The model under review builds one solid part; all positions refer to its coordinate system, in mm. A direction names the side the tool comes from. Coordinates: 2 decimals unless noted, no trailing zeros. Order: outer loops, then holes, each group sorted by start corner. A loop starts at its lowest first (then second) coordinate and runs counter-clockwise, first axis right, second up. Notation, with made-up numbers: (80.5, -28) -> (95.5, -28) arc R15 cw to (95.5, -10) -> close; hole circle Ø11 at (85, 44.25). An arc over 180 degrees is marked (long way). Use one line per item in the form item = value.
from build123d import *

# Parameters (mm, degrees)
F0_R     = 19
F0_R_2   = 17.5
F1_DEPTH = 30
F5_DEPTH = 2
F7_DEPTH = 8
F8_W     = 3.0304512245
F8_H     = 4
F8_W_2   = 3.9695487755
F9_DEPTH = 25


# Not quite as in the source:
# - a feature names something its author has since deleted; it is built from what else it names


with BuildPart() as f1:
    # F0 (on Top) → F1 (new body)
    with BuildSketch(Plane.XY):
        Circle(F0_R)
        Circle(F0_R_2, mode=Mode.SUBTRACT)
    extrude(amount=F1_DEPTH)

    # F2 (on Front) → F3 (revolve)
    with BuildSketch(Plane.XZ):
        with BuildLine():
            Line((0, 41.805047949), (0, 30))
            Line((0, 30), (19, 30))
            ThreePointArc((19, 30), (13.3813344534, 37.450646936), (5.1278058683, 41.805047949))
            Line((5.1278058683, 41.805047949), (0, 41.805047949))
        make_face()
    revolve(axis=Axis((0, 0, 35.9025239745), (0, 0, 1)))

    # F4 (on Top) → F5 (join)
    with BuildSketch(Plane.XY):
        with BuildLine():
            ThreePointArc((10, 0), (7.0710678119, -7.0710678119), (0, -10))
            Line((0, -10), (0, -19))
            ThreePointArc((0, -19), (13.4173031296, -13.4253390842), (18.972583327, 0))
            Line((18.972583327, 0), (10, 0))
        make_face()
    extrude(amount=F5_DEPTH)

    # F6 (on face) → F7 (join)
    with BuildSketch(Plane(origin=(0, 0, 0), x_dir=(1, 0, 0), z_dir=(0, 0, -1))):
        with BuildLine():
            Line((9.8692176419, 1.6119997323), (12.8996688664, 1.6119997323))
            ThreePointArc((12.8996688664, 1.6119997323), (8.6036039972, 9.745665614), (0, 13))
            Line((0, 13), (0, 10))
            ThreePointArc((0, 10), (6.4761100468, 7.6197111928), (9.8692176419, 1.6119997323))
        make_face()
    extrude(amount=F7_DEPTH)

    # F8 (on face) → F9 (cut)
    with BuildSketch(Plane(origin=(0, -1.6119997323, 0), x_dir=(-1, 0, 0), z_dir=(0, 1, 0))):
        with Locations((-11.3844432541, -2)):
            Rectangle(F8_W, F8_H)
        with Locations((-7.8844432541, -2)):
            Rectangle(F8_W_2, F8_H)
    extrude(amount=-F9_DEPTH, mode=Mode.SUBTRACT)


solid = f1.part
Item 1: Clearance check with flat-ended pins moving along their axes: pin 1 (10 mm diameter, centred on x = 7, y = -11, fed in from +Z); pin 2 (3.5 mm diameter, centred on x = 11, z = -5, fed in from +Y); pin 3 (6 mm diameter, centred on x = 8, z = 15, fed in from +Y). State where each tip first meets the part, or that it passes through.
Results found:
pin_1 = 40.78
pin_2 = -1.61
pin_3 = 18.33
Item 2: Draft analysis for pull direction X (two halves, no side actions). For faces 5 (the face through (7, -8, -8)), 6 (the face through (5.9, -10, -2)), 7 (the face through (0, 0, 30)), state which applies: released by +X, released by -X, zero draft, split by the parting line, or undercut.
Results found:
face_5 = zero draft
face_6 = released by +X
face_7 = undercut
Item 3: Tool access review of faces 1 (the face through (7.04, -10.93, -4.83)), 2 (the face through (9, -9, 2)), 3 (the face through (11, -1.612, -6)), 4 (the face through (14, 0, 1)): name each direction out of +Z, -Z, +X, -X, +Y, -Y from which nothing blocks a thin tool from reaching the whole face with its end or side.
Results found:
face_1 = -Z, +X, -Y
face_2 = none
face_3 = -Z, +X, -X, +Y
face_4 = -Z
Item 4: To check wall thickness, follow L1, parallel to X at y = 0, z = 19.25; L2, parallel to Z at x = 1, y = 2.5. State the ranges of each line that lie inside material, in increasing order. Write a range as from..to.
Results found:
L1 = -19..-17.5, 17.5..19
L2 = 30..41.81
Item 5: We need section A-A (z = 17.5). Write out the cut boundary in (x, y).
Results found:
outline = circle Ø38 at (0, 0); hole circle Ø35 at (0, 0)
